Design review of the part built by this model. Coordinates are the model's own, in mm. Give positions to 0.01 mm unless a question says otherwise; leave off trailing zeros. Order: outer loops, then holes, each group sorted by start corner. A loop starts at its lowest first (then second) coordinate and runs counter-clockwise, first axis right, second up. Notation, with made-up numbers: (29, 29.5) -> (79, 29.5) arc R23 ccw to (79, 41.5) -> close; hole circle Ø10 at (-24.5, 19.25). An arc over 180 degrees is marked (long way). Answer in a Markdown table with one row per item. Add a question column.
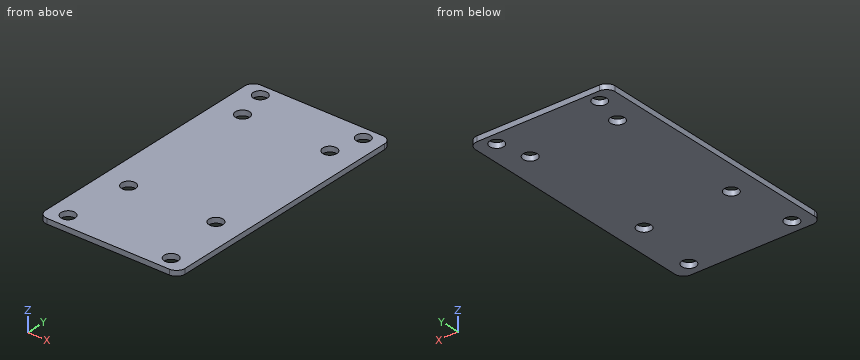
```python
from build123d import *

# Parameters (mm, degrees)
SKETCH1_W           = 80
SKETCH1_H           = 150
SKETCH1_R           = 4
BOSS_EXTRUDE1_DEPTH = 3
FILLET3_R           = 5


with BuildPart() as part:
    # Sketch1 → Boss-Extrude1 (new body)
    with BuildSketch(Plane.XY):
        Rectangle(SKETCH1_W, SKETCH1_H)
        with Locations((-29.5, 68)):
            Circle(SKETCH1_R, mode=Mode.SUBTRACT)
        with Locations((29.5, 68)):
            Circle(SKETCH1_R, mode=Mode.SUBTRACT)
        with Locations((29.5, -67)):
            Circle(SKETCH1_R, mode=Mode.SUBTRACT)
        with Locations((-29.5, -67)):
            Circle(SKETCH1_R, mode=Mode.SUBTRACT)
        with Locations((-25, 50)):
            Circle(SKETCH1_R, mode=Mode.SUBTRACT)
        with Locations((25, 50)):
            Circle(SKETCH1_R, mode=Mode.SUBTRACT)
        with Locations((25, -30)):
            Circle(SKETCH1_R, mode=Mode.SUBTRACT)
        with Locations((-25, -30)):
            Circle(SKETCH1_R, mode=Mode.SUBTRACT)
    extrude(amount=BOSS_EXTRUDE1_DEPTH)

    # Fillet3
    fillet3_edges = [part.edges().sort_by_distance(p)[0] for p in [
        (40, -75, 1.5),
        (-40, -75, 1.5),
        (-40, 75, 1.5),
        (40, 75, 1.5),
    ]]
    fillet(fillet3_edges, radius=FILLET3_R)


solid = part.part
```
1) Add section B-B, the plane z = 1.5. Give the number of separate pieces and of enclosed holes in the cut face, and give its area (3 significant figures).
2) Add section A-A, the plane y = -30. Write out the cut boundary in (x, z).
3) Clearance check with a flat-ended pin moving along its axis: P1, Ø5, axis at x = 25, y = -30, coming from the +Z side. State where the tip first meets the part, or that it passes through.
4) Add section C-C, the plane x = 23.5. Write out the cut boundary in (y, z), and give its area (3 significant figures).
5) For L1, parallel to Y at x = 29.5, z = 1.8; L2, parallel to Y at x = -25, z = 0.8; L3, parallel to X at y = 53.5, z = 1.2, list the stretches that pass through material, from the lowest coordinate up.
Verdict:
| question | item | result |
|---|---|---|
| 1 | separate pieces | 1 |
| 1 | enclosed holes | 8 |
| 1 | area | 11,600 mm2 |
| 2 | outline | (-40, 0) -> (-29, 0) -> (-29, 3) -> (-40, 3) -> close; (-21, 0) -> (21, 0) -> (21, 3) -> (-21, 3) -> close; (29, 0) -> (40, 0) -> (40, 3) -> (29, 3) -> close |
| 3 | P1 | passes through |
| 4 | outline | (-75, 0) -> (-33.71, 0) -> (-33.71, 3) -> (-75, 3) -> close; (-26.29, 0) -> (46.29, 0) -> (46.29, 3) -> (-26.29, 3) -> close; (53.71, 0) -> (75, 0) -> (75, 3) -> (53.71, 3) -> close |
| 4 | area | 406 mm2 |
| 5 | L1 | y = -75 to -71, -63 to 64, 72 to 75 |
| 5 | L2 | y = -75 to -34, -26 to 46, 54 to 75 |
| 5 | L3 | x = -40 to -26.94, -23.06 to 23.06, 26.94 to 40 |
